Part print with two shaded views. Sizes in mm from the minimum x, y, z corner. A direction names the side the tool comes from. Give positions to 0.01 mm unless a question says otherwise; leave off trailing zeros. Write each loop counter-clockwise with the first axis right and the second up, starting at its lowest first coordinate (ties: lowest second). Pieces come first, ordered by that corner, then holes.
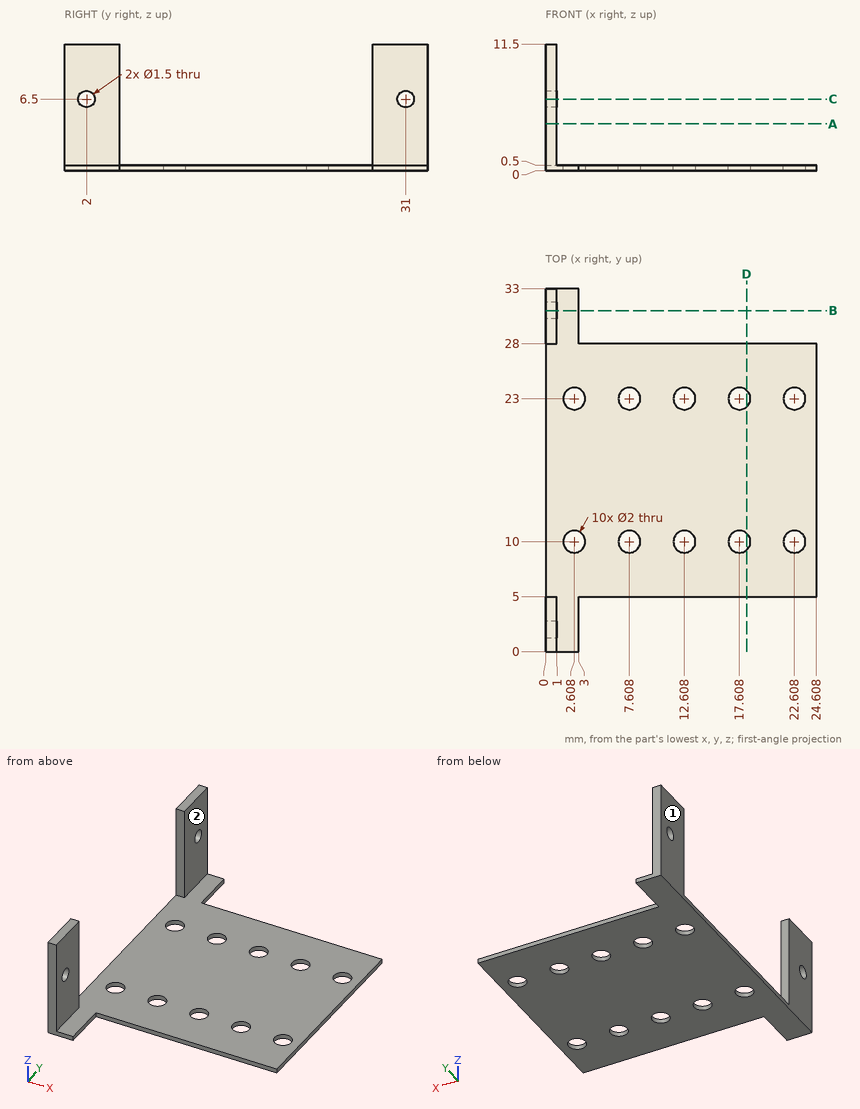
1) Saw through at D-D, the plane x = 18.25. Write the cut outline in (y, z).
Answers follow:
outline: (5, 0) - (9.23, 0) - (9.23, 0.5) - (5, 0.5) - close; (10.77, 0) - (22.23, 0) - (22.23, 0.5) - (10.77, 0.5) - close; (23.77, 0) - (28, 0) - (28, 0.5) - (23.77, 0.5) - close
2) Pin check, flat tips, straight feed: pin 1 Ø1.2 at (x, y) = (2.61, 23) entering from -Z; pin 2 Ø2 at (y, z) = (2, 6.5) entering from +X; pin 3 Ø2.5 at (x, y) = (17.61, 10) entering from +Z. Stop position of each tip, or through.
Answers follow:
pin 1: passes through
pin 2: stops at x = 1
pin 3: stops at z = 0.5
3) Saw through at B-B, the plane y = 31. Write the cut outline in (x, z).
Answers follow:
outline: (0, 0) - (3, 0) - (3, 0.5) - (1, 0.5) - (1, 5.75) - (0, 5.75) - close; (0, 7.25) - (1, 7.25) - (1, 11.5) - (0, 11.5) - close
4) Saw through at A-A, the plane z = 4.25. Write the cut outline in (x, y).
Answers follow:
outline: (0, 0) - (1, 0) - (1, 5) - (0, 5) - close; (0, 28) - (1, 28) - (1, 33) - (0, 33) - close
5) Wall check: L1, parallel to Z at x = 0.4, y = 2; L2, parallel to X at y = 4.5, z = 4.5; L3, parallel to Z at x = 17, y = 17.5. Give the ranges that are in metal, low to high.
Answers follow:
L1: z = 0 to 5.75, 7.25 to 11.5
L2: x = 0 to 1
L3: z = 0 to 0.5
6) Saw through at C-C, the plane z = 6.5. Write the cut outline in (x, y).
Answers follow:
outline: (0, 0) - (1, 0) - (1, 1.25) - (0, 1.25) - close; (0, 2.75) - (1, 2.75) - (1, 5) - (0, 5) - close; (0, 28) - (1, 28) - (1, 30.25) - (0, 30.25) - close; (0, 31.75) - (1, 31.75) - (1, 33) - (0, 33) - close
7) 3-axis set-ups, long thin cutter, end or side, ignore diameter. For the marked faces 1 and 2: which of +Z, -Z, +X, -X, +Y, -Y reach the whole face in a straight line?
Answers follow:
face 1: +Z, -Z, -X, +Y, -Y
face 2: +Z, +X, +Y, -Y
